Source: CAD feature listing. Evaluate the final solid. Frame: model axes, mm. A direction names the side the tool comes from. Round coordinates to 2 decimals unless told otherwise and drop trailing zeros. Loops run counter-clockwise (first coordinate to the right, second up) from the corner with the lowest first, then second, coordinate; pieces in that order, holes last. Notation, with made-up numbers: M 63,53 L 100,53 A19 ccw 100,59 Z; hole C -32,-38.75 d6. An arc over 180 degrees is marked long. One line per item, written item: value.
from build123d import *

# Parameters (mm, degrees)
SKETCH4_R          = 4.8514
SKETCH4_R_2        = 4.69265
CUT_EXTRUDE2_DEPTH = 4.064
CUT_EXTRUDE1_DEPTH = 4.064
CIRPATTERN1_COUNT  = 15
SKETCH6_R          = 1.5875
CUT_EXTRUDE3_DEPTH = 12.415131329


with BuildPart() as part:
    # Sketch1 → Revolve1 (revolve)
    with BuildSketch(Plane.XY, mode=Mode.PRIVATE) as revolve1_sk:
        with BuildLine():
            Line((-5.5626, 2.38125), (5.5626, 2.38125))
            Line((5.5626, 2.38125), (5.5626, 7.0485))
            Line((5.5626, 7.0485), (5.0419, 7.0485))
            ThreePointArc((5.0419, 7.0485), (4.654552953, 6.276378742), (4.5212, 5.4229))
            Line((4.5212, 5.4229), (4.5212, 4.8514))
            Line((4.5212, 4.8514), (0.4572, 4.8514))
            Line((0.4572, 4.8514), (0.4572, 5.9944))
            Line((0.4572, 5.9944), (-0.5969, 7.0485))
            Line((-0.5969, 7.0485), (-5.5626, 7.0485))
            Line((-5.5626, 7.0485), (-5.5626, 2.38125))
        make_face()
    revolve(revolve1_sk.sketch.rotate(Axis((-5.5626, 0, 0), (1, 0, 0)), 90), axis=Axis((-5.5626, 0, 0), (1, 0, 0)))

    # Sketch4 → Cut-Extrude2 (cut)
    with BuildSketch(Plane(origin=(0.4572, 0, 0), x_dir=(0, 0, -1), z_dir=(1, 0, 0))):
        Circle(SKETCH4_R)
        Circle(SKETCH4_R_2, mode=Mode.SUBTRACT)
    extrude(amount=CUT_EXTRUDE2_DEPTH, mode=Mode.SUBTRACT)

    # Sketch3 → Cut-Extrude1 (cut)
    with BuildSketch(Plane(origin=(0.4572, 0, 0), x_dir=(0, 0, -1), z_dir=(1, 0, 0))):
        with BuildLine():
            Line((-0.641825655, 4.648550726), (-0.344589457, 4.011125642))
            Line((-0.344589457, 4.011125642), (0.344589457, 4.011125642))
            Line((0.344589457, 4.011125642), (0.641825655, 4.648550726))
            ThreePointArc((0.641825655, 4.648550726), (0, 4.69265), (-0.641825655, 4.648550726))
        make_face()
    cut_extrude1 = extrude(amount=CUT_EXTRUDE1_DEPTH, mode=Mode.SUBTRACT)

    # CirPattern1: Cut-Extrude1 ×15 about axis
    cirpattern1_axis = Axis((0, 0, 0), (1, 0, 0))
    for i in range(1, CIRPATTERN1_COUNT):
        add(cut_extrude1.rotate(cirpattern1_axis, i * 360 / CIRPATTERN1_COUNT), mode=Mode.SUBTRACT)

    # Sketch6 → Cut-Extrude3 (cut, through all)
    with BuildSketch(Plane(origin=(0, 0, 0), x_dir=(1, 0, 0), z_dir=(0, 1, 0))):
        with Locations(Location((-2.5527, 0, 0), (0, 0, 90))):
            Circle(SKETCH6_R)
    extrude(amount=CUT_EXTRUDE3_DEPTH, mode=Mode.SUBTRACT)


solid = part.part
1. Pull-direction query (Y, two-part tool) for faces 4 (the face through (5.299, 6.253, 3.252)), 5 (the face through (0.08, -2.36, -0.31)), 6 (the face through (-5.563, 3, 0)); classes: released by +Y, released by -Y, zero draft, split by the parting line, or undercut.
Report:
face 4: split by the parting line
face 5: undercut
face 6: zero draft
2. Section query C-C (x = -2). Return the cut outline in (y, z).
Report:
outline: M 1.86,-1.49 A2.38 cw long 1.86,1.49 L 6.89,1.49 A7.05 ccw long 6.89,-1.49 Z
3. Pin query (flat end, axial travel): pin 1 (5 mm diameter, centred on x = -2.5, y = 4.5, fed in from +Z); pin 2 (4 mm diameter, centred on x = 2.5, y = 5, fed in from -Z); pin 3 (4 mm diameter, centred on x = 1, y = 2, fed in from +Z). Return the tip coordinate at first contact, or that it passes through.
Report:
pin 1: stops at z = 6.76
pin 2: stops at z = -3.03
pin 3: stops at z = 7
4. Section query A-A (z = 0). Return the cut outline in (x, y).
Report:
outline: M -5.56,-7.05 L -0.6,-7.05 L 0.46,-5.99 L 0.46,-4.69 L 4.52,-4.69 L 4.52,-5.42 A2.8 ccw 5.04,-7.05 L 5.56,-7.05 L 5.56,-2.38 L -5.56,-2.38 Z; M -5.56,2.38 L -4.14,2.38 L -4.14,7.05 L -5.56,7.05 Z; M -0.97,2.38 L 5.56,2.38 L 5.56,7.05 L 5.04,7.05 A2.8 ccw 4.52,5.42 L 4.52,4.01 L 0.46,4.01 L 0.46,5.99 L -0.6,7.05 L -0.97,7.05 Z
5. Ray query, line 1 (X direction, y = 2, z = -4.5); line 2 (Y direction, x = 0.75, z = 0); line 3 (X direction, y = 5.5, z = 0). Return the intervals inside material, ascending. Write a range as [from, to].
Report:
line 1: x = [-5.56, 0.46], [4.52, 5.56]
line 2: y = [-4.69, -2.38], [2.38, 4.01]
line 3: x = [-5.56, -4.14], [-0.97, 0.46], [4.52, 5.56]
6. Section query B-B (x = 0). Return the cut outline in (y, z).
Report:
outline: C 0,0 d12.9; hole C 0,0 d4.76
7. Reachability of faces 1 (the face through (-3.11, -6.99, -0.92)), 2 (the face through (0.457, 1.2, 4.1)), 3 (the face through (-1, 4.38, 0.34)) from +Z, -Z, +X, -X, +Y, -Y: full face, straight path, thin tool, end or side. Return the list, or none.
Report:
face 1: +X, -X
face 2: none
face 3: +Y
